Can you work these out from the model? Positions are in its coordinate system, mm. A direction names the side the tool comes from. Give positions to 0.01 mm unless a question says otherwise; leave off trailing zeros. Order: outer loops, then holes, each group sorted by start corner. A loop starts at its lowest first (then second) coordinate and runs counter-clockwise, first axis right, second up.
```python
from build123d import *

# Parameters (mm, degrees)
SZKIC1_W                    = 60
SZKIC1_H                    = 25
DODANIE_WYCI_GNI_CIE1_DEPTH = 1
DODANIE_WYCI_GNI_CIE2_DEPTH = 50
SZKIC4_R                    = 2
WYTNIJ_WYCI_GNI_CIE1_DEPTH  = 61
SZKIC5_W                    = 17
SZKIC5_H                    = 2
WYTNIJ_WYCI_GNI_CIE2_DEPTH  = 35
SZKIC6_W                    = 20
SZKIC6_H                    = 25
WYTNIJ_WYCI_GNI_CIE3_DEPTH  = 3
SZKIC7_W                    = 20
SZKIC7_H                    = 25
WYTNIJ_WYCI_GNI_CIE4_DEPTH  = 3
SFAZOWANIE1_SIZE            = 10
SZKIC8_R                    = 2.5
WYTNIJ_WYCI_GNI_CIE5_DEPTH  = 3
SZKIC9_W                    = 14
SZKIC9_H                    = 2
WYTNIJ_WYCI_GNI_CIE6_DEPTH  = 50


with BuildPart() as part:
    # Szkic1 → Dodanie-wyciągnięcie1 (new body)
    with BuildSketch(Plane.XY):
        with Locations((30, 12.5)):
            Rectangle(SZKIC1_W, SZKIC1_H)
    extrude(amount=DODANIE_WYCI_GNI_CIE1_DEPTH)

    # Szkic3 → Dodanie-wyciągnięcie2 (add)
    with BuildSketch(Plane.XY.offset(1)):
        Polygon((0, 0), (0, 25), (60, 25), (60, 0), (57, 0), (57, 23), (40, 23), (40, 0), (37, 0), (37, 23), (23, 23), (23, 0), (20, 0), (20, 23), (3, 23), (3, 0), align=None)
    extrude(amount=DODANIE_WYCI_GNI_CIE2_DEPTH)

    # Szkic4 → Wytnij-wyciągnięcie1 (cut, through all)
    with BuildSketch(Plane.ZY):
        with Locations((25, 12.5)):
            Circle(SZKIC4_R)
        with Locations((40, 12.5)):
            Circle(SZKIC4_R)
    extrude(amount=-WYTNIJ_WYCI_GNI_CIE1_DEPTH, mode=Mode.SUBTRACT)

    # Szkic5 → Wytnij-wyciągnięcie2 (cut)
    with BuildSketch(Plane.XY.offset(51)):
        with Locations((48.5, 24)):
            Rectangle(SZKIC5_W, SZKIC5_H)
        with Locations((11.5, 24)):
            Rectangle(SZKIC5_W, SZKIC5_H)
    extrude(amount=-WYTNIJ_WYCI_GNI_CIE2_DEPTH, mode=Mode.SUBTRACT)

    # Szkic6 → Wytnij-wyciągnięcie3 (cut)
    with BuildSketch(Plane.ZY):
        with Locations((41, 12.5)):
            Rectangle(SZKIC6_W, SZKIC6_H)
    extrude(amount=-WYTNIJ_WYCI_GNI_CIE3_DEPTH, mode=Mode.SUBTRACT)

    # Szkic7 → Wytnij-wyciągnięcie4 (cut)
    with BuildSketch(Plane(origin=(60, 0, 0), x_dir=(0, 0, -1), z_dir=(1, 0, 0))):
        with Locations((-41, 12.5)):
            Rectangle(SZKIC7_W, SZKIC7_H)
    extrude(amount=-WYTNIJ_WYCI_GNI_CIE4_DEPTH, mode=Mode.SUBTRACT)

    # Sfazowanie1
    sfazowanie1_edges = [part.edges().sort_by_distance(p)[0] for p in [
        (1.5, 0, 31),
        (58.5, 0, 31),
        (21.5, 0, 51),
        (38.5, 0, 51),
    ]]
    chamfer(sfazowanie1_edges, length=SFAZOWANIE1_SIZE)

    # Szkic8 → Wytnij-wyciągnięcie5 (cut)
    with BuildSketch(Plane.XY.offset(1)):
        with Locations((11.5, 11.5)):
            Circle(SZKIC8_R)
        with Locations((48.5, 11.5)):
            Circle(SZKIC8_R)
    extrude(amount=-WYTNIJ_WYCI_GNI_CIE5_DEPTH, mode=Mode.SUBTRACT)

    # Szkic9 → Wytnij-wyciągnięcie6 (cut)
    with BuildSketch(Plane.XY.offset(51)):
        with Locations((30, 24)):
            Rectangle(SZKIC9_W, SZKIC9_H)
    extrude(amount=-WYTNIJ_WYCI_GNI_CIE6_DEPTH, mode=Mode.SUBTRACT)


solid = part.part
```
1) Suppose I cut it at C-C (y = 5). Please give me the cut outline in (x, z), and give its area (3 significant figures).
2) Suppose I cut it at B-B (x = 11.5). Please give me the cut outline in (y, z).
3) We'd pull the mould along Y, two halves only. Please class faces 1 (the face through (39, 0, 14)), 2 (the face through (50.81, 10.54, 0.51)), 3 (the face through (38.479, 14.483, 39.74)), 4 (the face through (48, 24, 16)): +Y half, -Y half, draft (parallel to the pull), parting line (faces both ways), or undercut.
4) I'm going to push flat-ended pins straight in: pin 1 Ø3.5 at (x, y) = (1.5, 19.5) entering from +Z; pin 2 Ø6.5 at (x, y) = (48.5, 11.5) entering from -Z; pin 3 Ø8 at (x, y) = (27.5, 8.5) entering from +Z; pin 4 Ø5 at (x, z) = (32.5, 32.5) entering from +Y. Where does each tip first touch, or does it pass through?
5) If I drill on line 1 (X direction, y = 15.25, z = 10); line 2 (X direction, y = 21.5, z = 42); line 3 (Y direction, x = 20.85, z = 25), over which ranges is the centre line in solid material (lowest first)?
6) Suppose I cut it at D-D (z = 40). Please give me the cut outline in (x, y).
7) Which directions (+Z, -Z, +X, -X, +Y, -Y) give clear straight access to the entire face, cutting with the end or side of a thin tool? Please do faces 5 (the face through (49, 23, 8)), 6 (the face through (59, 17, 31)), 7 (the face through (59, 5, 26)), 8 (the face through (37, 15, 26)).
8) Suppose I cut it at A-A (z = 34.5). Please give me the cut outline in (x, y).
Results:
1. outline: (0, 0) - (60, 0) - (60, 26) - (57, 26) - (57, 1) - (40, 1) - (40, 46) - (37, 46) - (37, 1) - (23, 1) - (23, 46) - (20, 46) - (20, 1) - (3, 1) - (3, 26) - (0, 26) - close
1. area: 480 mm2
2. outline: (0, 0) - (9, 0) - (9, 1) - (0, 1) - close; (14, 0) - (25, 0) - (25, 16) - (23, 16) - (23, 1) - (14, 1) - close
3. face 1: -Y half
3. face 2: undercut
3. face 3: undercut
3. face 4: draft
4. pin 1: stops at z = 31
4. pin 2: stops at z = 0
4. pin 3: stops at z = 1
4. pin 4: passes through
5. line 1: x = 0 to 3, 20 to 23, 37 to 40, 57 to 60
5. line 2: x = 20 to 23, 37 to 40
5. line 3: y = 0 to 10.5, 14.5 to 25
6. outline: (20, 0) - (23, 0) - (23, 10.5) - (20, 10.5) - close; (20, 14.5) - (23, 14.5) - (23, 25) - (20, 25) - close; (37, 0) - (40, 0) - (40, 10.5) - (37, 10.5) - close; (37, 14.5) - (40, 14.5) - (40, 25) - (37, 25) - close
7. face 5: +Z, -Y
7. face 6: +Z, +X, +Y, -Y
7. face 7: +Z, +X, -Y
7. face 8: +Z, +Y, -Y
8. outline: (20, 0) - (23, 0) - (23, 25) - (20, 25) - close; (37, 0) - (40, 0) - (40, 25) - (37, 25) - close
